```python
from build123d import *

# Parameters (mm, degrees)
SKETCH1_R           = 4
BOSS_EXTRUDE1_DEPTH = 4
SKETCH2_R           = 7.75
SKETCH2_R_2         = 0.65
BOSS_EXTRUDE2_DEPTH = 6
SKETCH3_R           = 4
BOSS_EXTRUDE3_DEPTH = 4
CUT_EXTRUDE1_DEPTH  = 24


with BuildPart() as part:
    # Sketch1 → Boss-Extrude1 (new body)
    with BuildSketch(Plane(origin=(0, 0, 0), x_dir=(1, 0, 0), z_dir=(0, 1, 0))):
        with Locations(Location((0, 0, 0), (0, 0, 270))):
            Circle(SKETCH1_R)
    extrude(amount=BOSS_EXTRUDE1_DEPTH)

    # Sketch2 → Boss-Extrude2 (add)
    with BuildSketch(Plane(origin=(0, 4, 0), x_dir=(1, 0, 0), z_dir=(0, 1, 0))):
        with Locations(Location((0, 0, 0), (0, 0, 270))):
            Circle(SKETCH2_R)
        with Locations(Location((0, 6, 0), (0, 0, 270))):
            Circle(SKETCH2_R_2, mode=Mode.SUBTRACT)
        with Locations(Location((6, 0, 0), (0, 0, 270))):
            Circle(SKETCH2_R_2, mode=Mode.SUBTRACT)
        with Locations(Location((0, -6, 0), (0, 0, 270))):
            Circle(SKETCH2_R_2, mode=Mode.SUBTRACT)
        with Locations(Location((-6, 0, 0), (0, 0, 270))):
            Circle(SKETCH2_R_2, mode=Mode.SUBTRACT)
    extrude(amount=BOSS_EXTRUDE2_DEPTH)

    # Sketch3 → Boss-Extrude3 (add)
    with BuildSketch(Plane(origin=(0, 10, 0), x_dir=(1, 0, 0), z_dir=(0, 1, 0))):
        with Locations(Location((0, 0, 0), (0, 0, 270))):
            Circle(SKETCH3_R)
    extrude(amount=BOSS_EXTRUDE3_DEPTH)

    # Sketch4 → Cut-Extrude1 (cut)
    with BuildSketch(Plane(origin=(0, 14, 0), x_dir=(1, 0, 0), z_dir=(0, 1, 0))):
        Polygon((0, 2.5), (2.165063509, -1.25), (-2.165063509, -1.25), align=None)
    extrude(amount=-CUT_EXTRUDE1_DEPTH, mode=Mode.SUBTRACT)


solid = part.part
```
Verification items for the finished model (mm, model axes). A direction names the side the tool comes from. Coordinates: 2 decimals unless noted, no trailing zeros. Loops run counter-clockwise (first coordinate to the right, second up) from the corner with the lowest first, then second, coordinate; pieces in that order, holes last. Notation, with made-up numbers: (75.5, -3) -> (84.5, -3) arc R20 cw to (84.5, 34) -> close; hole circle Ø9 at (50.5, 86). An arc over 180 degrees is marked (long way). Put each result on its own line as item: value.
1. Section check D-D, the plane z = 2.5. Record the boundary of the cut face in (x, y), then the cut area to 3 significant figures.
Result set:
outline: (-7.34, 4) -> (-3.12, 4) -> (-3.12, 0) -> (3.12, 0) -> (3.12, 4) -> (7.34, 4) -> (7.34, 10) -> (3.12, 10) -> (3.12, 14) -> (-3.12, 14) -> (-3.12, 10) -> (-7.34, 10) -> close
area: 138 mm^2
2. Section check B-B, the plane x = -6. Record the boundary of the cut face in (y, z), then the cut area to 3 significant figures.
Result set:
outline: (4, -4.91) -> (10, -4.91) -> (10, -0.65) -> (4, -0.65) -> close; (4, 0.65) -> (10, 0.65) -> (10, 4.91) -> (4, 4.91) -> close
area: 51.1 mm^2
3. Mould release check, pull along Z, two halves, no side actions. Record for faces 1 (the face through (-3, 10, 3)), 2 (the face through (0, 7, 1.25)), 3 (the face through (7.684, 6.958, -1.009)): pulls with the +Z half, pulls with the -Z half, needs draft (parallel to the pull), parting line crosses it, or undercut.
Result set:
face 1: needs draft
face 2: undercut
face 3: parting line crosses it
4. Gauge pin test, flat ends, axial feed: P1, Ø6, axis at y = 7.5, z = 2, coming from the -X side; P2, Ø1.5, axis at x = 0, z = 6, coming from the +Y side; P3, Ø1.7, axis at x = 6, z = 0, coming from the -Y side; P4, Ø1.5, axis at y = 9, z = -5, coming from the -X side. Record the tip position at first contact, or that the pin passes through.
Result set:
P1: stops at x = -7.75
P2: stops at y = 10
P3: stops at y = 4
P4: stops at x = -6.48
5. Thickness scan on line 1 (X direction, y = 7.75, z = 0); line 2 (Y direction, x = -2, z = -6.25); line 3 (Z direction, x = 6.25, y = 4.5). Record the ranges inside material, lowest first.
Result set:
line 1: x = -7.75 to -6.65, -5.35 to -1.44, 1.44 to 5.35, 6.65 to 7.75
line 2: y = 4 to 10
line 3: z = -4.58 to -0.6, 0.6 to 4.58
6. Section check C-C, the plane z = 6. Record the boundary of the cut face in (x, y), then the cut area to 3 significant figures.
Result set:
outline: (-4.91, 4) -> (-0.65, 4) -> (-0.65, 10) -> (-4.91, 10) -> close; (0.65, 4) -> (4.91, 4) -> (4.91, 10) -> (0.65, 10) -> close
area: 51.1 mm^2
7. Section check A-A, the plane y = 4.75. Record the boundary of the cut face in (x, z).
Result set:
outline: circle Ø15.5 at (0, 0); hole circle Ø1.3 at (-6, 0); hole (-2.17, 1.25) -> (0, -2.5) -> (2.17, 1.25) -> close; hole circle Ø1.3 at (0, -6); hole circle Ø1.3 at (0, 6); hole circle Ø1.3 at (6, 0)
8. Tool access check on faces 4 (the face through (-3, 4, 3)), 5 (the face through (-3.905, 11.972, -0.867)), 6 (the face through (0, 0, 2)), 7 (the face through (-1.098, 7.098, -0.599)), 8 (the face through (0, 14, 2)). Record the directions out of +Z, -Z, +X, -X, +Y, -Y that give a thin tool (end or side, any length) a straight path to the whole face; none if there is none.
Result set:
face 4: -Y
face 5: +Y
face 6: +Z, -Z, +X, -X, -Y
face 7: +Y, -Y
face 8: +Z, -Z, +X, -X, +Y
